Source: three-view drawing plus pictorial views. Frame: mm from the lowest corner of the part. A direction names the side the tool comes from. Give positions to 0.01 mm unless a question says otherwise; leave off trailing zeros. Order: outer loops, then holes, each group sorted by start corner. A loop starts at its lowest first (then second) coordinate and runs counter-clockwise, first axis right, second up.
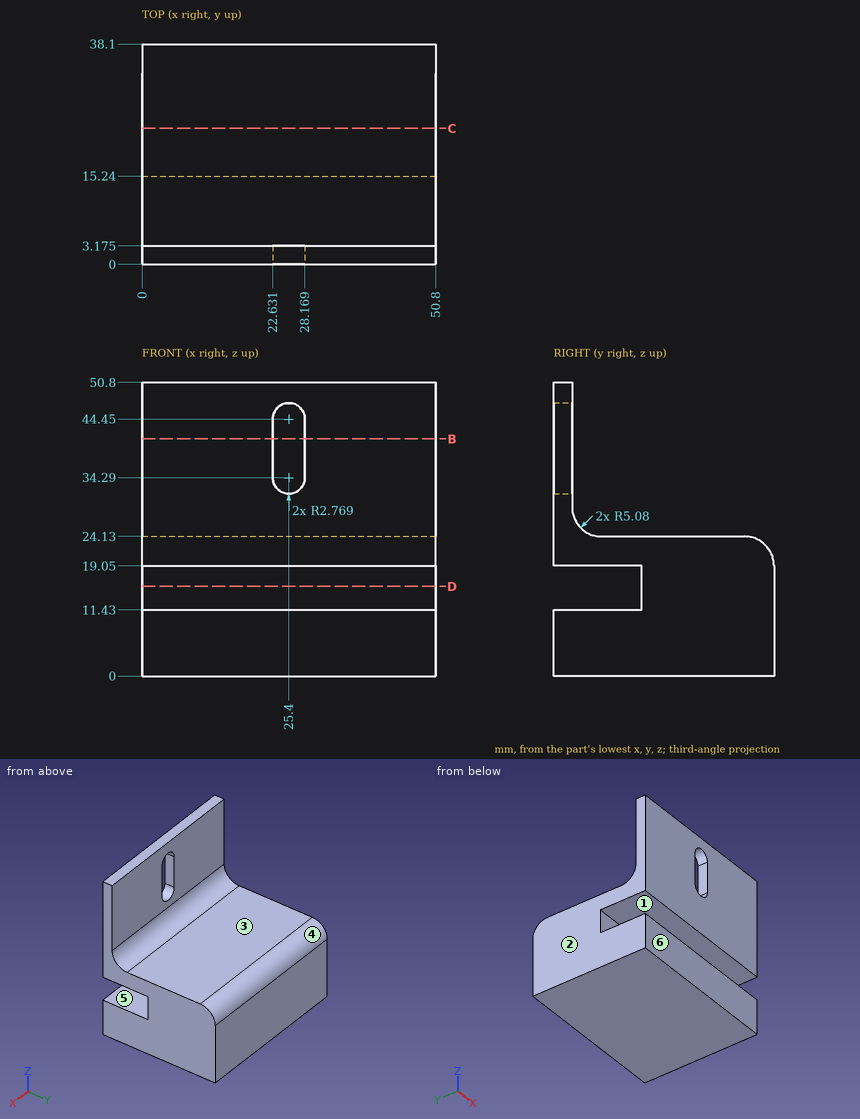
1) Ray query, L1, parallel to Z at x = 10, y = 14; L2, parallel to Z at x = 42, y = 28; L3, parallel to Y at x = 25, z = 18. Return the intervals inside material, ascending.
Checks:
L1: z = 0 to 11.43, 19.05 to 24.13
L2: z = 0 to 24.13
L3: y = 15.24 to 38.1
2) Section query C-C on y = 23.5. Output: boundary loops of the cut face in (x, z).
Checks:
outline: (0, 0) - (50.8, 0) - (50.8, 24.13) - (0, 24.13) - close
3) First-contact query: pin 1 Ø7.5 at (x, y) = (34, 18) entering from +Z; pin 2 Ø2 at (x, z) = (45, 45) entering from +Y (3 decimals); pin 3 Ø4 at (x, y) = (40, 6) entering from +Z (1 decimal). Flat tips, straight axial feed; report the tip coordinate or a pass-through.
Checks:
pin 1: stops at z = 24.13
pin 2: stops at y = 3.175
pin 3: stops at z = 26.4
4) Section query B-B on z = 41. Output: boundary loops of the cut face in (x, y) (1 decimal).
Checks:
outline: (0, 0) - (22.6, 0) - (22.6, 3.2) - (0, 3.2) - close; (28.2, 0) - (50.8, 0) - (50.8, 3.2) - (28.2, 3.2) - close
5) Pull-direction query (Z, two-part tool) for the marked faces 4, 5 and 6; classes: +Z half, -Z half, draft (parallel to the pull), parting line (faces both ways), or undercut.
Checks:
face 4: +Z half
face 5: undercut
face 6: draft
6) Section query D-D on z = 15.5. Output: boundary loops of the cut face in (x, y).
Checks:
outline: (0, 15.24) - (50.8, 15.24) - (50.8, 38.1) - (0, 38.1) - close
7) Reachability of the marked faces 1, 2 and 3 from +Z, -Z, +X, -X, +Y, -Y: full face, straight path, thin tool, end or side. Return the list, or none.
Checks:
face 1: +X, -X, -Y
face 2: +Z, -Z, -X, +Y, -Y
face 3: +Z, +X, -X, +Y
